Work out the finished part from the listing and answer in its coordinate system (mm). Face numbers are marked on the shaded views. A direction names the side the tool comes from. Round coordinates to 2 decimals unless told otherwise and drop trailing zeros. Write each loop counter-clockwise with the first axis right and the second up, starting at its lowest first coordinate (ties: lowest second). Pieces come first, ordered by that corner, then holes. Notation, with made-up numbers: (34.25, 30) -> (92.25, 30) arc R23 cw to (92.25, 54) -> close; hole circle Ø4 at (1.25, 9). An arc over 180 degrees is marked (long way). One line per item, written item: value.
```python
from build123d import *


with BuildPart() as part:
    # Sweep2: sweep along a path in Sketch1
    with BuildLine(Plane.XY) as sweep2_path:
        Line((-190.884848485, 85.898181818), (-89.284848485, 85.898181818))
        ThreePointArc((-89.284848485, 85.898181818), (20.963569163, 44.75210076), (77.296784563, -58.564318182))
    # Sketch2 → Sweep2 (sweep)
    with BuildSketch(Plane(origin=(-190.884848485, 0, 0), x_dir=(0, 0, -1), z_dir=(1, 0, 0))):
        Polygon((-63.5, 85.898181818), (63.5, 85.898181818), (63.5, 87.485681818), (44.45, 87.485681818), (44.45, 86.691931818), (-44.45, 86.691931818), (-44.45, 87.485681818), (-63.5, 87.485681818), align=None)
    sweep(path=sweep2_path.line)


solid = part.part
```
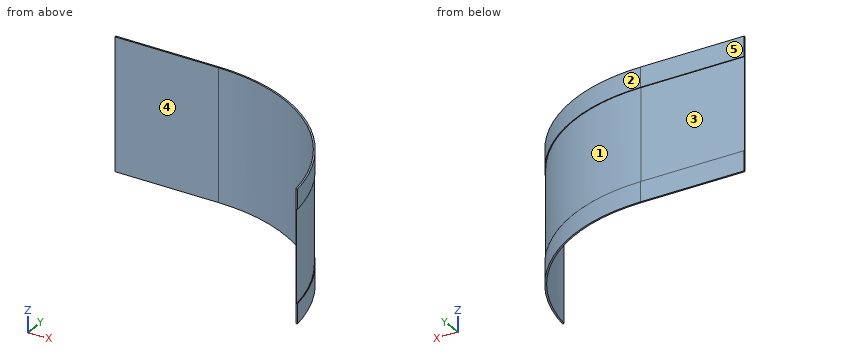
(1) Flat-ended cylindrical pins translate along their axes: pin 1 Ø3 at (x, z) = (-35.5, -23) entering from -Y; pin 2 Ø3 at (y, z) = (52, 34) entering from -X; pin 3 Ø8 at (x, z) = (23.5, 1) entering from +Y. Find the tip coordinate at first contact, or state that the pin passes through.
Reported:
pin 1: stops at y = 76.56
pin 2: stops at x = 9.98
pin 3: stops at y = 47.05
(2) Find section A-A on x = -4.5. Give the vertices of the cut face in (y, z).
Reported:
outline: (62.98, -63.5) -> (64.81, -63.5) -> (64.81, -44.45) -> (63.9, -44.45) -> (63.9, 44.45) -> (64.81, 44.45) -> (64.81, 63.5) -> (62.98, 63.5) -> close
(3) Consider probe 1 along Y at (x, z) = (-158.5, 3); probe 2 along X at (y, z) = (-11, -32.5); probe 3 along Y at (x, z) = (17, -57). Determine where each line is inside the solid, lowest interval first.
Reported:
probe 1: y = 85.9 to 86.69
probe 2: x = 63.1 to 63.98
probe 3: y = 48.08 to 50.13
(4) A tool of negligible diameter and unlimited length cuts with its end or side. For the marked faces 3, 4 and 5, from which of +Z, -Z, +X, -X, +Y, -Y can it reach the whole face along a straight path? Write none if from no direction.
Reported:
face 3: +X, -X, +Y
face 4: +Z, -Z, -X, -Y
face 5: +Z, -Z, +X, -X, +Y
(5) For a pull along Z with two mould halves and no side action, classify the marked faces 1 and 2 as pulls with the +Z half, pulls with the -Z half, needs draft (parallel to the pull), parting line crosses it, or undercut.
Reported:
face 1: undercut
face 2: needs draft
(6) Find section B-B on y = -27. Give the vertices of the cut face in (x, z).
Reported:
outline: (69.62, -63.5) -> (71.3, -63.5) -> (71.3, -44.45) -> (70.46, -44.45) -> (70.46, 44.45) -> (71.3, 44.45) -> (71.3, 63.5) -> (69.62, 63.5) -> close
